The model under review builds one solid part; all positions refer to its coordinate system, in mm. A direction names the side the tool comes from. Round coordinates to 2 decimals unless told otherwise and drop trailing zeros. Order: outer loops, then holes, each group sorted by start corner. A loop starts at its lowest first (then second) coordinate and runs counter-clockwise, first axis right, second up. Notation, with made-up numbers: (-21.75, 37) -> (-3.75, 37) arc R26 cw to (-3.75, 60) -> close; hole circle Ø7 at (77.25, 62). An arc over 180 degrees is marked (long way). Use a Markdown table: item, result. Add a question column.
```python
from build123d import *

# Parameters (mm, degrees)
SKETCH1_R           = 42.8625
SKETCH1_R_2         = 22.225
BOSS_EXTRUDE1_DEPTH = 3.175
CUT_EXTRUDE1_DEPTH  = 61.699822384
CUT_EXTRUDE3_DEPTH  = 61.699822384
FILLET1_R           = 2.54


with BuildPart() as part:
    # Sketch1 → Boss-Extrude1 (new body)
    with BuildSketch(Plane(origin=(0, 0, 0), x_dir=(1, 0, 0), z_dir=(0, 1, 0))):
        with Locations(Location((0, 0, 0), (0, 0, 270))):
            Circle(SKETCH1_R)
        with Locations(Location((0, 0, 0), (0, 0, 270))):
            Circle(SKETCH1_R_2, mode=Mode.SUBTRACT)
    extrude(amount=BOSS_EXTRUDE1_DEPTH)

    # Sketch2 → Cut-Extrude1 (cut, through all)
    with BuildSketch(Plane(origin=(0, 3.175, 0), x_dir=(1, 0, 0), z_dir=(0, 1, 0))):
        with BuildLine():
            ThreePointArc((19.39925, 33.600486629), (14.194693212, 32.20592984), (15.58925, 27.001373052))
            ThreePointArc((15.58925, 27.001373052), (0, -31.1785), (-15.58925, 27.001373052))
            ThreePointArc((-15.58925, 27.001373052), (-14.194693212, 32.20592984), (-19.39925, 33.600486629))
            ThreePointArc((-19.39925, 33.600486629), (0, -38.7985), (19.39925, 33.600486629))
        make_face()
    extrude(amount=-CUT_EXTRUDE1_DEPTH, mode=Mode.SUBTRACT)

    # Sketch6 → Cut-Extrude3 (cut, through all)
    with BuildSketch(Plane(origin=(0, 3.175, 0), x_dir=(1, 0, 0), z_dir=(0, 1, 0))):
        with BuildLine():
            Line((-21.34992109, -22.721789799), (-16.03711988, -22.721789799))
            ThreePointArc((-16.03711988, -22.721789799), (-15.390384879, -22.850433389), (-14.84210942, -23.216779339))
            Line((-14.84210942, -23.216779339), (-11.16498954, -26.893899219))
            ThreePointArc((-11.16498954, -26.893899219), (-10.61671408, -27.260245169), (-9.96997908, -27.388888759))
            Line((-9.96997908, -27.388888759), (9.96997908, -27.388888759))
            ThreePointArc((9.96997908, -27.388888759), (10.61671408, -27.260245169), (11.16498954, -26.893899219))
            Line((11.16498954, -26.893899219), (14.84210942, -23.216779339))
            ThreePointArc((14.84210942, -23.216779339), (15.390384879, -22.850433389), (16.03711988, -22.721789799))
            Line((16.03711988, -22.721789799), (21.34992109, -22.721789799))
            ThreePointArc((21.34992109, -22.721789799), (0, -31.1785), (-21.34992109, -22.721789799))
        make_face()
        with BuildLine():
            Line((29.1, -5.51000025), (29.1, 5.51000025))
            ThreePointArc((29.1, 5.51000025), (29.448279688, 6.53756368), (30.349569945, 7.14160111))
            ThreePointArc((30.349569945, 7.14160111), (31.1785, 0), (30.349569945, -7.14160111))
            ThreePointArc((30.349569945, -7.14160111), (29.448279688, -6.53756368), (29.1, -5.51000025))
        make_face()
        with BuildLine():
            Line((-29.1, 5.51000025), (-29.1, -5.51000025))
            ThreePointArc((-29.1, -5.51000025), (-29.448279688, -6.53756368), (-30.349569945, -7.14160111))
            ThreePointArc((-30.349569945, -7.14160111), (-31.1785, 0), (-30.349569945, 7.14160111))
            ThreePointArc((-30.349569945, 7.14160111), (-29.448279688, 6.53756368), (-29.1, 5.51000025))
        make_face()
    extrude(amount=-CUT_EXTRUDE3_DEPTH, mode=Mode.SUBTRACT)

    # Fillet1
    fillet1_edges = [part.edges().sort_by_distance(p)[0] for p in [
        (-30.349569945, 1.5875, 7.14160111),
        (-30.349569945, 1.5875, -7.14160111),
        (21.34992109, 1.5875, 22.721789799),
        (-21.34992109, 1.5875, 22.721789799),
        (30.349569945, 1.5875, -7.14160111),
        (30.349569945, 1.5875, 7.14160111),
    ]]
    fillet(fillet1_edges, radius=FILLET1_R)


solid = part.part
```
Q1. Add section D-D (y = 2). State how many separate pieces and enclosed holes the cut face has, then the cut area to 3 significant figures.
Q2. Add section A-A (z = 0). Write out the cut boundary in (x, y) (1 decimal).
Q3. Wall thickness on line 1 (X direction, y = 2.55, z = 0) (1 decimal); line 2 (X direction, y = 1.9, z = -13); line 3 (Z direction, x = 10.5, y = 0.3): over which ranges is each line inside the solid? List them lowest first. Write a range as [from, to].
Q4. Insertion check: pin 1 (1.5 mm diameter, centred on y = 1.5, z = 4, fed in from +X); pin 2 (1.6 mm diameter, centred on x = 5, y = 1.5, fed in from +Z). Each pin has a flat end and moves straight along its axis. Give the tip position at first contact, or say it passes through.
Q5. Add section B-B (x = 0). Write out the cut boundary in (y, z) (1 decimal), then the cut area to 3 significant figures.
Q6. Machinability: for faces 1 (the flat face through (3.4, 0, -22.4)), 2 (the cylindrical face through (-26.77, 1.61, 15.98)), which of the approach directions +Z, -Z, +X, -X, +Y, -Y give a long, thin tool a straight path to every point of the face, cutting with its end or side? Answer none if there is none.
Q7. Mouldability with a two-part tool opening along Z and no side actions: class faces 3 (the cylindrical face through (-26.1, 1.6, -34)), 4 (the cylindrical face through (26.88, 1.61, 15.8)), 5 (the flat face through (3.4, 3.175, -22.4)) as pulls with the +Z half, pulls with the -Z half, needs draft (parallel to the pull), parting line crosses it, or undercut.
Q8. Add section C-C (z = 33.5). Write out the cut boundary in (x, y) (3 decimals), then the cut area to 3 significant figures.
Report:
| question | item | result |
|---|---|---|
| 1 | separate pieces | 1 |
| 1 | enclosed holes | 2 |
| 1 | area | 2,600 mm² |
| 2 | outline | (-42.9, 0) -> (-38.8, 0) -> (-38.8, 3.2) -> (-42.9, 3.2) -> close; (-29.1, 0) -> (-22.2, 0) -> (-22.2, 3.2) -> (-29.1, 3.2) -> close; (22.2, 0) -> (29.1, 0) -> (29.1, 3.2) -> (22.2, 3.2) -> close; (38.8, 0) -> (42.9, 0) -> (42.9, 3.2) -> (38.8, 3.2) -> close |
| 3 | line 1 | x = [-42.9, -38.8], [-29.1, -22.2], [22.2, 29.1], [38.8, 42.9] |
| 3 | line 2 | x = [-40.84, -36.56], [-28.34, -18.03], [18.03, 28.34], [36.56, 40.84] |
| 3 | line 3 | z = [-41.56, -19.59], [19.59, 27.3], [37.35, 41.56] |
| 4 | pin 1 | stops at x = 42.74 |
| 4 | pin 2 | stops at z = 42.66 |
| 5 | outline | (0, -42.9) -> (3.2, -42.9) -> (3.2, -22.2) -> (0, -22.2) -> close; (0, 22.2) -> (3.2, 22.2) -> (3.2, 27.4) -> (0, 27.4) -> close; (0, 38.8) -> (3.2, 38.8) -> (3.2, 42.9) -> (0, 42.9) -> close |
| 5 | area | 94.8 mm² |
| 6 | face 1 | +Z, -Z, +X, -X, -Y |
| 6 | face 2 | +Y, -Y |
| 7 | face 3 | parting line crosses it |
| 7 | face 4 | undercut |
| 7 | face 5 | needs draft |
| 8 | outline | (-26.738, 0) -> (-19.572, 0) -> (-19.572, 3.175) -> (-26.738, 3.175) -> close; (19.572, 0) -> (26.738, 0) -> (26.738, 3.175) -> (19.572, 3.175) -> close |
| 8 | area | 45.5 mm² |
